Here's how the part is built. I have some questions about the finished solid (model axes, mm). Face numbers are marked on the shaded views. A direction names the side the tool comes from. Round coordinates to 2 decimals unless told otherwise and drop trailing zeros. Order: outer loops, then holes, each group sorted by start corner. A loop starts at its lowest first (then second) coordinate and runs counter-clockwise, first axis right, second up. Notation, with made-up numbers: (-29, 69.25) - (24, 69.25) arc R17 ccw to (24, 90.25) - close; hole circle Ø11 at (56.25, 51). An arc over 180 degrees is marked (long way). Answer as a JSON object with one key per item and string values.
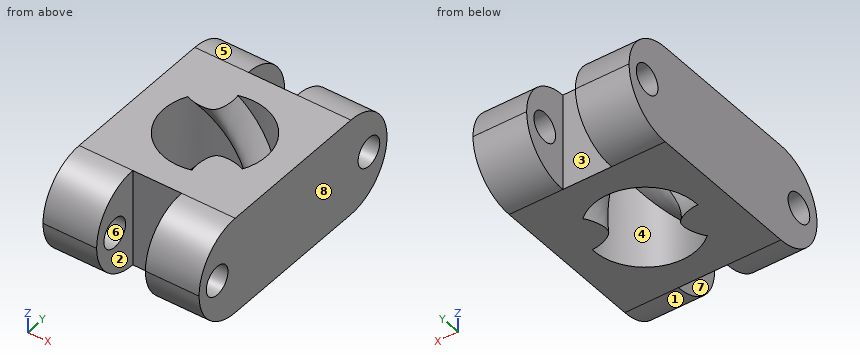
Autodesk Inventor part; units mm, degrees
ref_plane "YZ Plane" through (0, 0, 0) normal (1, 0, 0) x (0, 1, 0)
ref_plane "XZ Plane" through (0, 0, 0) normal (0, 1, 0) x (-1, 0, 0)
ref_plane "XY Plane" through (0, 0, 0) normal (0, 0, 1) x (1, 0, 0)
sketch "Sketch1" plane through (0, 0, 0) normal (0, 0, 1) x (1, 0, 0)
  circle A0 centre (0, 0) radius 5.25
  line L0 (0, 0) -> (-8, 0)
  line L1 (-8, 0) -> (-8, 8)
  line L2 (-8, 8) -> (8, 8)
  line L3 (8, 8) -> (8, -8)
  line L4 (8, -8) -> (-8, -8)
  line L5 (-8, -8) -> (-8, 0)
  line L6 (0, -8) -> (-2.5, -8)
  line L7 (-2.5, -8) -> (-2.5, -13)
  line L8 (-2.5, -13) -> (-8, -13)
  line L9 (-8, -13) -> (-8, -8)
  line L10 (0, -8) -> (2.5, -8)
  line L11 (2.5, -8) -> (2.5, -13)
  line L12 (2.5, -13) -> (8, -13)
  line L13 (8, -13) -> (8, -8)
  line L14 (8, 0) -> (8, -2.5)
  line L15 (8, 0) -> (8, 2.5)
  line L16 (13, -2.5) -> (13, -8)
  line L17 (13, -8) -> (8, -8)
  line L18 (13, 2.5) -> (13, 8)
  line L19 (13, 8) -> (8, 8)
  line L20 (8, 2.5) -> (13, 2.5)
  line L21 (8, -2.5) -> (13, -2.5)
  line L22 (8, 8) -> (8, -8)
  line L23 (0, 8) -> (2.5, 8)
  line L24 (0, 8) -> (-2.5, 8)
  line L25 (2.5, 13) -> (8, 13)
  line L26 (8, 13) -> (8, 8)
  line L27 (-2.5, 13) -> (-8, 13)
  line L28 (-8, 13) -> (-8, 8)
  line L29 (-2.5, 8) -> (-2.5, 13)
  line L30 (2.5, 8) -> (2.5, 13)
  line L31 (-8, 8) -> (8, 8)
  line L32 (-8, 0) -> (-8, 2.5)
  line L33 (-8, 0) -> (-8, -2.5)
  line L34 (-13, 2.5) -> (-13, 8)
  line L35 (-13, 8) -> (-8, 8)
  line L36 (-13, -2.5) -> (-13, -8)
  line L37 (-13, -8) -> (-8, -8)
  line L38 (-8, -2.5) -> (-13, -2.5)
  line L39 (-8, 2.5) -> (-13, 2.5)
  line L40 (-8, -8) -> (-8, 8)
  dimension "d0" = 10.5
  dimension "d1" = 8
  dimension "d2" = 8
  dimension "d3" = 16
  dimension "d4" = 16
  dimension "d5" = 16
  dimension "d33" = 2.5
  dimension "d34" = 5
  dimension "d35" = 2.5
  dimension "d38" = 360
extrude "Extrusion1" add sketch "Sketch1" along normal blind 10 contours L1 L2 L3 L4 L5 | L28 L27 L29 L2 | L4 L7 L8 L9 | L30 L25 L26 L2 | L4 L13 L12 L11
ref_plane "Work Plane1" through (-8, 0, 0) normal (0, -1, 0) x (1, 0, 0)
sketch "Sketch3" plane through (-8, 0, 0) normal (0, -1, 0) x (1, 0, 0)
  line L0 (13.3034, 0) -> (13.3034, -2.5)
  line L1 (2.75, 0) -> (2.75, 10)
  line L2 (2.75, 0) -> (2.75, -2.5)
  circle A0 centre (13.3034, -2.5) radius 2.25
  circle A1 centre (2.75, -2.5) radius 2.25
  point P0 (8, 0)
  dimension "d9" = 2.5
  dimension "d10" = 2.5
  dimension "d11" = 4.5
  dimension "d12" = 4.5
coil "Coil1" sketch "Sketch3" operation add axis through (0, 0, -10) along (0, 0, 1) pitch 35 turns 1 hand right contours A1
coil "Coil2" sketch "Sketch3" operation add axis through (0, 0, -10) along (0, 0, 1) pitch 35 turns 1 hand right contours A0
sketch "Sketch4" plane through (-8, -8, 0) normal (0, -1, 0) x (1, 0, 0)
  line L0 (10.5, 10) -> (5.5, 10)
  line L1 (0, 10) -> (16, 10)
  line L2 (16, 10) -> (16, 40)
  line L3 (16, 40) -> (0, 40)
  line L4 (0, 40) -> (0, 10)
  line L5 (10.5, 0) -> (5.5, 0)
  line L6 (0, 0) -> (16, 0)
  line L7 (16, 0) -> (16, -15)
  line L8 (16, -15) -> (0, -15)
  line L9 (0, -15) -> (0, 0)
  point P0 (8, 0)
  point P1 (16, 0)
  dimension "d29" = 30
  dimension "d30" = 15
extrude "Extrusion2" cut sketch "Sketch4" against normal through all
fillet "Fillet1" radius 5 8 edges at (5.25, -13, 10) (-5.25, -13, 10) (-5.25, 13, 10) (5.25, 13, 10) (-5.25, 13, 0) (5.25, 13, 0) (-5.25, -13, 0) (5.25, -13, 0)
sketch "Sketch6" plane through (8, -8, 0) normal (1, 0, 0) x (0, 0, -1)
  arc A0 (-10, 0) -> (0, 0) centre (-5, 0) ccw
  line L0 (-5, -5) -> (-5, -2.5)
  circle A1 centre (-5, -2.5) radius 1.5
  arc A2 (0, 16) -> (-10, 16) centre (-5, 16) ccw
  line L1 (-5, 21) -> (-5, 18.5)
  circle A3 centre (-5, 18.5) radius 1.5
  point P0 (0, 8)
  dimension "d41" = 2.5
  dimension "d42" = 3
  dimension "d43" = 2.5
  dimension "d44" = 3
extrude "Extrusion3" cut sketch "Sketch6" against normal through all
equation "\"d2\" = d1"
equation "\"d3\" = 2 * d1"
equation "\"d4\" = d3"
equation "\"d5\" = d3"
properties part number "screw_nut"
1. For the marked faces 1, 2, 3, 4 and 5, which set-ups out of +Z, -Z, +X, -X, +Y, -Y let a thin tool reach every point of the face, with its end or its side?
Responses:
{"face 1": "-Z, +X, -X, -Y", "face 2": "+Z, -Z, -Y", "face 3": "+Z, -Z, +Y", "face 4": "none", "face 5": "+Z, +X, -X, +Y"}
2. For P1, Ø4, axis at x = -1, z = 3, coming from the -Y side; P2, Ø4, axis at x = 5.5, z = 1, coming from the +Y side; P3, Ø2, axis at x = 1, z = 1.5, coming from the -Y side, each with a flat end and sliding along its axis, tell me the tip position at first contact or that it passes through.
Responses:
{"P1": "y = -12.95", "P2": "y = 12.58", "P3": "y = -8"}
3. Imagine slicing it at A-A (x = -6.25). Give the number of separate pieces and of enclosed holes in the cut face, plus the area to 3 significant figures.
Responses:
{"separate pieces": "1", "enclosed holes": "2", "area": "224 mm2"}
4. If I drill on L1, parallel to X at y = -4, z = 4.75 (3 decimals); L2, parallel to X at y = 0, z = 2.5; L3, parallel to X at y = 8.75, z = 1.25, over which ranges is the centre line in solid material (lowest first)? Write a range as [from, to].
Responses:
{"L1": "[-8, -3.4], [-3.185, 0.271], [3.4, 8]", "L2": "[-8, -5.25], [5.25, 8]", "L3": "[-8, -2.5], [2.5, 8]"}
5. Thinking about a two-plate mould opening in X: for the marked faces 6, 7 and 8, which applies, pulls with the +X half, pulls with the -X half, needs draft (parallel to the pull), parting line crosses it, or undercut?
Responses:
{"face 6": "needs draft", "face 7": "undercut", "face 8": "pulls with the +X half"}
6. Imagine slicing it at B-B (y = -10.5). List the corners of the cut face in (x, z) for me, plus the area to 3 significant figures.
Responses:
{"outline": "(-8, 0.67) - (-2.5, 0.67) - (-2.5, 3.5) - (-8, 3.5) - close; (-8, 6.5) - (-2.5, 6.5) - (-2.5, 9.33) - (-8, 9.33) - close; (2.5, 0.67) - (8, 0.67) - (8, 3.5) - (2.5, 3.5) - close; (2.5, 6.5) - (8, 6.5) - (8, 9.33) - (2.5, 9.33) - close", "area": "62.3 mm2"}
